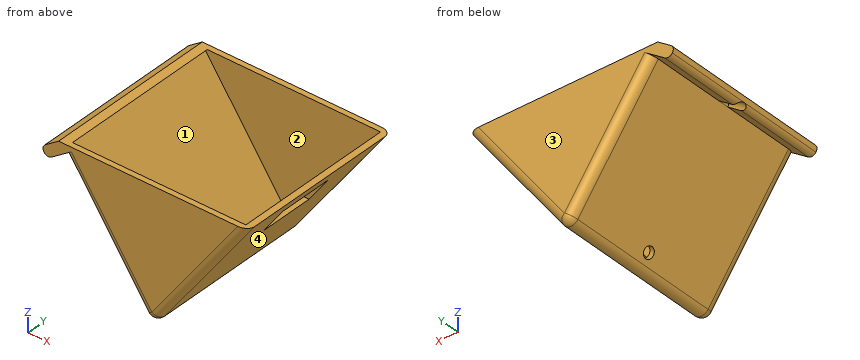
from build123d import *

# Parameters (mm, degrees)
EXTRUDE_1_DEPTH     = 32
EXTRUDE_2_DEPTH     = 32
CUT_EXTRUDE_1_DEPTH = 4
SHELL_START         = 1
SHELL_1_DEPTH       = 30
CUT_EXTRUDE_START   = 27.611157
SKETCH_4_W          = 5
SKETCH_4_H          = 10
CUT_EXTRUDE_2_DEPTH = 4.85474
CUT_EXTRUDE_3_REACH = 55.413
SKETCH_6_R          = 1
FILLET_1_R          = 1
FILLET_2_R          = 1
FILLET_3_R          = 1.5


# Read off the part's stored shape, not the designer's step: 抽壳1
with BuildPart() as part:
    # 草图1 → 凸台-拉伸1 (new body)
    with BuildSketch(Plane(origin=(0, 0, 0), x_dir=(1, 0, 0), z_dir=(0, 1, 0))):
        Polygon((0, 0), (35, 0), (17.207293091, 24.574561329), align=None)
    extrude(amount=EXTRUDE_1_DEPTH)

    # 草图2 → 凸台-拉伸2 (add)
    with BuildSketch(Plane(origin=(0, 0, 0), x_dir=(1, 0, 0), z_dir=(0, 1, 0))):
        Polygon((0, 0), (-3.276608177, 2.294305745), (-2.129455304, 3.932609834), (1.147152873, 1.638304089), align=None)
    extrude(amount=EXTRUDE_2_DEPTH)

    # 草图3 → 切除-拉伸1 (cut)
    with BuildSketch(Plane(origin=(-3.276608177, 0, -2.294305745), x_dir=(-0.5735764363510533, 0, 0.8191520442889868), z_dir=(-0.8191520442889868, 0, -0.5735764363510533))):
        with BuildLine():
            Line((-2, 17), (-2, 15))
            ThreePointArc((-2, 15), (-1, 16), (-2, 17))
        make_face()
    extrude(amount=-CUT_EXTRUDE_1_DEPTH, mode=Mode.SUBTRACT)

    # 抽壳1 outline → 抽壳1 (cut)
    with BuildSketch(Plane(origin=(0, 0, 0), x_dir=(1, 0, 0), z_dir=(0, 1, 0)).offset(SHELL_START)):
        Polygon((1.392728481, 0.245575608), (1.743446796, 0), (33.76540748, 0), (17.220918494, 22.850573626), align=None)
    extrude(amount=SHELL_1_DEPTH, mode=Mode.SUBTRACT)

    # 草图4 → 切除-拉伸2 (cut)
    with BuildSketch(Plane(origin=(0, 0, 0), x_dir=(0, 0, -1), z_dir=(1, 0, 0)).offset(CUT_EXTRUDE_START)):
        with Locations((6, 16)):
            Rectangle(SKETCH_4_W, SKETCH_4_H)
    extrude(amount=CUT_EXTRUDE_2_DEPTH, mode=Mode.SUBTRACT)

    # 草图6 → 切除-拉伸3 (cut, up to next)
    with BuildSketch(Plane(origin=(0, 0, 0), x_dir=(-0.5735764363510502, 0, 0.819152044288989), z_dir=(-0.819152044288989, 0, -0.5735764363510502)), mode=Mode.PRIVATE) as cut_extrude_3_sk1:
        with Locations((-26, 16)):
            Circle(SKETCH_6_R)
    cut_extrude_3_tool1 = extrude(cut_extrude_3_sk1.sketch, amount=-CUT_EXTRUDE_3_REACH, mode=Mode.PRIVATE) & part.part
    add(cut_extrude_3_tool1.solids().sort_by_distance((14.912987, 16, -21.297953))[0], mode=Mode.SUBTRACT)

    # 圆角1
    fillet_1_edges = [part.edges().sort_by_distance(p)[0] for p in [
        (-2.129455304, 24.5, -3.932609834),
        (-2.129455304, 7.5, -3.932609834),
    ]]
    fillet(fillet_1_edges, radius=FILLET_1_R - 0.0001)  # a hair under: the kernel refuses the full size

    # 圆角2
    fillet_2_edges = [part.edges().sort_by_distance(p)[0] for p in [
        (-3.276608177, 16, -2.294305745),
    ]]
    fillet(fillet_2_edges, radius=FILLET_2_R - 0.0001)  # a hair under: the kernel refuses the full size

    # 圆角3
    fillet_3_edges = [part.edges().sort_by_distance(p)[0] for p in [
        (26.103646545, 32, -12.287280664),
        (26.103646545, 0, -12.287280664),
        (9.177222982, 32, -13.106432709),
        (9.177222982, 0, -13.106432709),
        (17.207293091, 16, -24.574561329),
    ]]
    fillet(fillet_3_edges, radius=FILLET_3_R)


solid = part.part
For this review, take the finished solid that the model builds, in its own axes (mm). Face numbers are marked on the shaded views. Round coordinates to 2 decimals unless told otherwise and drop trailing zeros. Use a Markdown table: item, result. Add a question column.
Item 1: Mouldability with a two-part tool opening along X and no side actions: class the marked faces 1, 2, 3 and 4 as released by +X, released by -X, zero draft, split by the parting line, or undercut.
Item 2: Insertion check: pin 1 (1.5 mm diameter, centred on x = 10.5, y = 6.5, fed in from -Z); pin 2 (8 mm diameter, centred on x = 8, y = 12, fed in from -Z); pin 3 (2 mm diameter, centred on y = 6.5, z = -16, fed in from -X). Each pin has a flat end and moves straight along its axis. Give the tip position at first contact, or say it passes through.
Item 3: To check wall thickness, follow line 1 along Y through (x, z) = (24.5, -2); line 2 along X through (y, z) = (21, -20); line 3 along X through (y, z) = (5, -0.75). State the ranges of each line that lie inside material, in increasing order.
Geometry results:
| question | item | result |
|---|---|---|
| 1 | face 1 | undercut |
| 1 | face 2 | undercut |
| 1 | face 3 | zero draft |
| 1 | face 4 | released by +X |
| 2 | pin 1 | stops at z = -16.07 |
| 2 | pin 2 | stops at z = -17.14 |
| 2 | pin 3 | stops at x = 10.5 |
| 3 | line 1 | y = 0 to 1, 31 to 32 |
| 3 | line 2 | x = 14 to 15.22, 19.28 to 20.52 |
| 3 | line 3 | x = -1.07 to 1.75, 33.22 to 34.46 |
